from build123d import *

# Parameters (mm, degrees)
SKETCH2_R           = 1.6
BOSS_EXTRUDE1_DEPTH = 4
CUT_EXTRUDE1_DEPTH  = 2
CUT_EXTRUDE2_DEPTH  = 1.5
SKETCH6_R           = 1.5
CUT_EXTRUDE3_DEPTH  = 52.039200621
BOSS_EXTRUDE4_START = 1.5
SKETCH7_R           = 4
SKETCH7_R_2         = 1.5
BOSS_EXTRUDE4_DEPTH = 1.5
CIRPATTERN1_COUNT   = 4
FILLET2_R           = 2
FILLET4_R           = 30


with BuildPart() as part:
    # Sketch2 → Boss-Extrude1 (new body)
    with BuildSketch(Plane(origin=(0, 0, 0), x_dir=(1, 0, 0), z_dir=(0, 1, 0))):
        Polygon((-12.5, 35), (12.5, 35), (23.334523779, 36.062445841), (36.062445841, 23.334523779), (35, 12.5), (35, -12.5), (36.062445841, -23.334523779), (23.334523779, -36.062445841), (12.5, -35), (-12.5, -35), (-23.334523779, -36.062445841), (-36.062445841, -23.334523779), (-35, -12.5), (-35, 12.5), (-36.062445841, 23.334523779), (-23.334523779, 36.062445841), align=None)
        with Locations(Location((22.627416998, 31.112698372, 0), (0, 0, 270))):
            Circle(SKETCH2_R, mode=Mode.SUBTRACT)
        with Locations(Location((31.112698372, 22.627416998, 0), (0, 0, 270))):
            Circle(SKETCH2_R, mode=Mode.SUBTRACT)
        with Locations(Location((22.627416998, -31.112698372, 0), (0, 0, 270))):
            Circle(SKETCH2_R, mode=Mode.SUBTRACT)
        with Locations(Location((31.112698372, -22.627416998, 0), (0, 0, 270))):
            Circle(SKETCH2_R, mode=Mode.SUBTRACT)
        with Locations(Location((-31.112698372, -22.627416998, 0), (0, 0, 270))):
            Circle(SKETCH2_R, mode=Mode.SUBTRACT)
        with Locations(Location((-22.627416998, -31.112698372, 0), (0, 0, 270))):
            Circle(SKETCH2_R, mode=Mode.SUBTRACT)
        with Locations(Location((-22.627416998, 31.112698372, 0), (0, 0, 270))):
            Circle(SKETCH2_R, mode=Mode.SUBTRACT)
        with Locations(Location((-31.112698372, 22.627416998, 0), (0, 0, 270))):
            Circle(SKETCH2_R, mode=Mode.SUBTRACT)
    extrude(amount=BOSS_EXTRUDE1_DEPTH)

    # Sketch4 → Cut-Extrude1 (cut)
    with BuildSketch(Plane(origin=(0, 4, 0), x_dir=(1, 0, 0), z_dir=(0, 1, 0))):
        Polygon((29, 12.012193309), (12.012193309, 29), (-12.012193309, 29), (-29, 12.012193309), (-29, -12.012193309), (-12.012193309, -29), (12.012193309, -29), (29, -12.012193309), align=None)
    extrude(amount=-CUT_EXTRUDE1_DEPTH, mode=Mode.SUBTRACT)

    # Sketch5 → Cut-Extrude2 (cut)
    with BuildSketch(Plane(origin=(0, 2, 0), x_dir=(1, 0, 0), z_dir=(0, 1, 0))):
        with BuildLine():
            Line((-24.816214135, 10.215498353), (-16.816214135, 6.779959319))
            ThreePointArc((-16.816214135, 6.779959319), (-15.494869505, 5.673946029), (-15, 4.023394242))
            Line((-15, 4.023394242), (-15, -4.023394242))
            ThreePointArc((-15, -4.023394242), (-15.494869505, -5.673946029), (-16.816214135, -6.779959319))
            Line((-16.816214135, -6.779959319), (-24.816214135, -10.215498353))
            ThreePointArc((-24.816214135, -10.215498353), (-27.650551787, -9.964063771), (-29, -7.458933276))
            Line((-29, -7.458933276), (-29, 7.458933276))
            ThreePointArc((-29, 7.458933276), (-27.650551787, 9.964063771), (-24.816214135, 10.215498353))
        make_face()
        with BuildLine():
            Line((10.215498353, 24.816214135), (6.779959319, 16.816214135))
            ThreePointArc((6.779959319, 16.816214135), (5.673946029, 15.494869505), (4.023394242, 15))
            Line((4.023394242, 15), (-4.023394242, 15))
            ThreePointArc((-4.023394242, 15), (-5.673946029, 15.494869505), (-6.779959319, 16.816214135))
            Line((-6.779959319, 16.816214135), (-10.215498353, 24.816214135))
            ThreePointArc((-10.215498353, 24.816214135), (-9.964063771, 27.650551787), (-7.458933276, 29))
            Line((-7.458933276, 29), (7.458933276, 29))
            ThreePointArc((7.458933276, 29), (9.964063771, 27.650551787), (10.215498353, 24.816214135))
        make_face()
        with BuildLine():
            Line((24.816214135, -10.215498353), (16.816214135, -6.779959319))
            ThreePointArc((16.816214135, -6.779959319), (15.494869505, -5.673946029), (15, -4.023394242))
            Line((15, -4.023394242), (15, 4.023394242))
            ThreePointArc((15, 4.023394242), (15.494869505, 5.673946029), (16.816214135, 6.779959319))
            Line((16.816214135, 6.779959319), (24.816214135, 10.215498353))
            ThreePointArc((24.816214135, 10.215498353), (27.650551787, 9.964063771), (29, 7.458933276))
            Line((29, 7.458933276), (29, -7.458933276))
            ThreePointArc((29, -7.458933276), (27.650551787, -9.964063771), (24.816214135, -10.215498353))
        make_face()
        with BuildLine():
            Line((-10.215498353, -24.816214135), (-6.779959319, -16.816214135))
            ThreePointArc((-6.779959319, -16.816214135), (-5.673946029, -15.494869505), (-4.023394242, -15))
            Line((-4.023394242, -15), (4.023394242, -15))
            ThreePointArc((4.023394242, -15), (5.673946029, -15.494869505), (6.779959319, -16.816214135))
            Line((6.779959319, -16.816214135), (10.215498353, -24.816214135))
            ThreePointArc((10.215498353, -24.816214135), (9.964063771, -27.650551787), (7.458933276, -29))
            Line((7.458933276, -29), (-7.458933276, -29))
            ThreePointArc((-7.458933276, -29), (-9.964063771, -27.650551787), (-10.215498353, -24.816214135))
        make_face()
    extrude(amount=-CUT_EXTRUDE2_DEPTH, mode=Mode.SUBTRACT)

    # Sketch6 → Cut-Extrude3 (cut, through all)
    with BuildSketch(Plane(origin=(0, 2, 0), x_dir=(1, 0, 0), z_dir=(0, 1, 0))):
        with Locations(Location((15.25, 15.25, 0), (0, 0, 270))):
            Circle(SKETCH6_R)
    cut_extrude3 = extrude(amount=-CUT_EXTRUDE3_DEPTH, mode=Mode.SUBTRACT)

    # Sketch7 → Boss-Extrude4 (add)
    with BuildSketch(Plane(origin=(0, 2, 0), x_dir=(1, 0, 0), z_dir=(0, 1, 0)).offset(BOSS_EXTRUDE4_START)):
        with Locations(Location((15.25, 15.25, 0), (0, 0, 270))):
            Circle(SKETCH7_R)
        with Locations(Location((15.25, 15.25, 0), (0, 0, 270))):
            Circle(SKETCH7_R_2, mode=Mode.SUBTRACT)
    boss_extrude4 = extrude(amount=-BOSS_EXTRUDE4_DEPTH)

    # CirPattern1: Cut-Extrude3, Boss-Extrude4 ×4 about axis
    cirpattern1_axis = Axis((0, 0, 0), (0, 1, 0))
    add([cut_extrude3.rotate(cirpattern1_axis, i * 360 / CIRPATTERN1_COUNT) for i in range(1, CIRPATTERN1_COUNT)], mode=Mode.SUBTRACT)
    add([boss_extrude4.rotate(cirpattern1_axis, i * 360 / CIRPATTERN1_COUNT) for i in range(1, CIRPATTERN1_COUNT)])

    # Fillet2
    # the kernel refuses this fillet: 2 mm, written as the material it adds along each edge
    with BuildSketch(Plane(origin=(15.25, 2, -15.25), x_dir=(0, 0, 1), z_dir=(-1, 0, 0))) as fillet2_piece_1:
        with BuildLine():
            CenterArc((5.936491673, 2), FILLET2_R, 194.477512186, 75.522487814)
            Line((4, 1.5), (3.961270167, 1.49))
            ThreePointArc((3.961270167, 1.49), (3.96, 0.75), (3.96, 0))
            Line((3.96, 0), (4, -0.04))
            Line((4, -0.04), (5.936491673, -0.04))
            Line((5.936491673, -0.04), (5.936491673, 0))
        make_face()
    revolve(axis=Axis((15.25, 2, -15.25), (0, 1, 0)))
    with BuildSketch(Plane(origin=(15.25, 2, 15.25), x_dir=(-1, 0, 0), z_dir=(0, 0, -1))) as fillet2_piece_2:
        with BuildLine():
            CenterArc((5.936491673, 2), FILLET2_R, 194.477512186, 75.522487814)
            Line((4, 1.5), (3.961270167, 1.49))
            ThreePointArc((3.961270167, 1.49), (3.96, 0.75), (3.96, 0))
            Line((3.96, 0), (4, -0.04))
            Line((4, -0.04), (5.936491673, -0.04))
            Line((5.936491673, -0.04), (5.936491673, 0))
        make_face()
    revolve(axis=Axis((15.25, 2, 15.25), (0, 1, 0)))
    with BuildSketch(Plane(origin=(-15.25, 2, 15.25), x_dir=(0, 0, -1), z_dir=(1, 0, 0))) as fillet2_piece_3:
        with BuildLine():
            CenterArc((5.936491673, 2), FILLET2_R, 194.477512186, 75.522487814)
            Line((4, 1.5), (3.961270167, 1.49))
            ThreePointArc((3.961270167, 1.49), (3.96, 0.75), (3.96, 0))
            Line((3.96, 0), (4, -0.04))
            Line((4, -0.04), (5.936491673, -0.04))
            Line((5.936491673, -0.04), (5.936491673, 0))
        make_face()
    revolve(axis=Axis((-15.25, 2, 15.25), (0, 1, 0)))
    with BuildSketch(Plane(origin=(-15.25, 2, -15.25), x_dir=(1, 0, 0), z_dir=(0, 0, 1))) as fillet2_piece_4:
        with BuildLine():
            CenterArc((5.936491673, 2), FILLET2_R, 194.477512186, 75.522487814)
            Line((4, 1.5), (3.961270167, 1.49))
            ThreePointArc((3.961270167, 1.49), (3.96, 0.75), (3.96, 0))
            Line((3.96, 0), (4, -0.04))
            Line((4, -0.04), (5.936491673, -0.04))
            Line((5.936491673, -0.04), (5.936491673, 0))
        make_face()
    revolve(axis=Axis((-15.25, 2, -15.25), (0, 1, 0)))

    # Fillet4
    # the kernel refuses this fillet: 30 mm, written as the material it adds along each edge
    with BuildSketch(Plane(origin=(35, 0, -12.5), x_dir=(0.09759304388629828, 0, -0.9952264052892723), z_dir=(0, 1, 0)), Plane(origin=(35, 0, 12.5), x_dir=(0, 0, -1), z_dir=(0, 1, 0)), Plane(origin=(12.5, 0, 35), x_dir=(0.9952264052892723, 0, 0.09759304388629875), z_dir=(0, 1, 0)), Plane(origin=(12.5, 0, -35), x_dir=(-1, 0, 0), z_dir=(0, 1, 0))) as fillet4_piece_1:
        with BuildLine():
            CenterArc((FILLET4_R * 0.0489132680019, -FILLET4_R), FILLET4_R, 90, 5.600584003)
            Line((-FILLET4_R * 0.0486797758844, -FILLET4_R * 0.00477359471073), (0, 0))
            Line((0, 0), (FILLET4_R * 0.0489132680019, 0))
        make_face()
    extrude(amount=4)
    with BuildSketch(Plane(origin=(-12.5, 0, 35), x_dir=(-0.9952264052892463, 0, 0.09759304388656506), z_dir=(0, 1, 0)), Plane(origin=(-35, 0, 12.5), x_dir=(0, 0, -1), z_dir=(0, 1, 0)), Plane(origin=(-35, 0, -12.5), x_dir=(-0.09759304388656435, 0, -0.9952264052892463), z_dir=(0, 1, 0)), Plane(origin=(-12.5, 0, -35), x_dir=(1, 0, 0), z_dir=(0, 1, 0))) as fillet4_piece_2:
        with BuildLine():
            CenterArc((FILLET4_R * 0.048913268002, FILLET4_R), FILLET4_R, 264.399415997, 5.600584003)
            Line((-FILLET4_R * 0.0486797758846, FILLET4_R * 0.00477359471075), (0, 0))
            Line((0, 0), (FILLET4_R * 0.048913268002, 0))
        make_face()
    extrude(amount=4)


solid = part.part
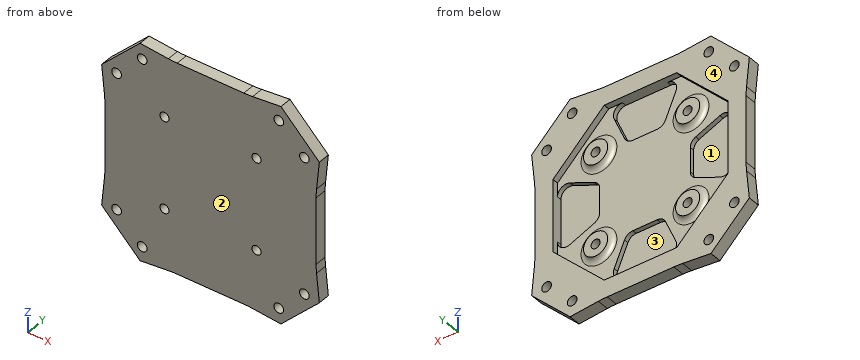
The model under review builds one solid part; all positions refer to its coordinate system, in mm. Face numbers are marked on the shaded views. A direction names the side the tool comes from. Round coordinates to 2 decimals unless told otherwise and drop trailing zeros. Loops run counter-clockwise (first coordinate to the right, second up) from the corner with the lowest first, then second, coordinate; pieces in that order, holes last. Notation, with made-up numbers: (73, 3.5) - (92, 3.5) arc R35 cw to (92, 36.5) - close; hole circle Ø2 at (88.5, 27.5). An arc over 180 degrees is marked (long way). Use CSV: the item, a comma, the result in double quotes.
(1) Clearance check with flat-ended pins moving along their axes: P1, Ø4, axis at x = 15.25, z = -15.25, coming from the -Y side; P2, Ø2.5, axis at x = -16.5, z = 15.5, coming from the +Y side; P3, Ø2, axis at y = 2.5, z = 15.5, coming from the +X side; P4, Ø1.9, axis at x = -31.11, z = 22.63, coming from the -Y side. State where each tip first meets the part, or that it passes through.
Working result:
P1,"stops at y = 0"
P2,"stops at y = 3.5"
P3,"stops at x = 35.39"
P4,"passes through"
(2) Take a section at C-C, the plane z = -28. Give the boundary of the cut face in (x, y) (3 decimals).
Working result:
outline,"(-31.397, 0) - (31.397, 0) - (31.397, 4) - (13.012, 4) - (13.012, 2) - (9.695, 2) - (9.695, 0.5) - (-9.695, 0.5) - (-9.695, 2) - (-13.012, 2) - (-13.012, 4) - (-31.397, 4) - close"
(3) Take a section at A-A, the plane z = -1. Give the boundary of the cut face in (x, y).
Working result:
outline,"(-35, 0) - (35, 0) - (35, 4) - (29, 4) - (29, 0.5) - (15, 0.5) - (15, 2) - (-15, 2) - (-15, 0.5) - (-29, 0.5) - (-29, 4) - (-35, 4) - close"
(4) For line 1 (Z direction, x = -30, y = 1.65); line 2 (X direction, y = 2.4, z = -5), list the stretches that pass through material, from the lowest coordinate up.
Working result:
line 1,"z = -29.4 to -23.78, -21.48 to 21.48, 23.78 to 29.4"
line 2,"x = -35 to -29, 29 to 35"
(5) Take a section at B-B, the plane y = 1.25. State how many separate pieces and enclosed holes the cut face has, plus the area to 3 significant figures.
Working result:
separate pieces,"1"
enclosed holes,"16"
area,"3,670 mm^2"
(6) The part is to be moulded in two halves that separate along Z. For the marked faces 3 and 4, say which applies: pulls with the +Z half, pulls with the -Z half, needs draft (parallel to the pull), parting line crosses it, or undercut.
Working result:
face 3,"undercut"
face 4,"needs draft"
(7) Machinability: for the marked faces 1 and 2, which of the approach directions +Z, -Z, +X, -X, +Y, -Y give a long, thin tool a straight path to every point of the face, cutting with its end or side? Answer none if there is none.
Working result:
face 1,"+Y"
face 2,"+Z, -Z, +X, -X, -Y"
